Design review of the part built by this model. Coordinates are the model's own, in mm. Face numbers are marked on the shaded views. A direction names the side the tool comes from. Round coordinates to 2 decimals unless told otherwise and drop trailing zeros. Order: outer loops, then holes, each group sorted by start corner. A loop starts at its lowest first (then second) coordinate and runs counter-clockwise, first axis right, second up.
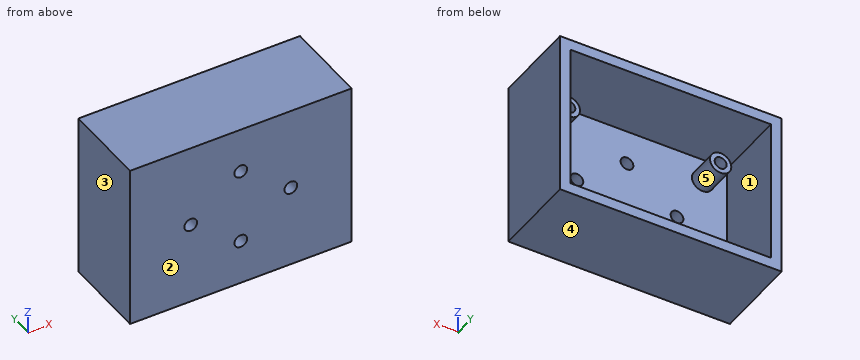
from build123d import *

# Parameters (mm, degrees)
SKETCH_1_W          = 52
SKETCH_1_H          = 39
SKETCH_1_W_2        = 47
SKETCH_1_H_2        = 34
EXTRUDE_1_DEPTH     = 20
SKETCH_2_R          = 2.5
EXTRUDE_2_DEPTH     = 10
EXTRUDE_2_2_DEPTH   = 10
EXTRUDE_2_3_DEPTH   = 10
EXTRUDE_2_4_DEPTH   = 10
SKETCH_3_R          = 1.4
CUT_EXTRUDE_1_DEPTH = 7
SKETCH_4_W          = 52
SKETCH_4_H          = 39
EXTRUDE_3_DEPTH     = 3
SKETCH_5_R          = 1.5
CUT_EXTRUDE_2_DEPTH = 37.67764987


with BuildPart() as part:
    # Sketch 1 → Extrude 1 (new body)
    with BuildSketch(Plane(origin=(0, 0, 0), x_dir=(1, 0, 0), z_dir=(0, 1, 0))):
        Rectangle(SKETCH_1_W, SKETCH_1_H)
        Rectangle(SKETCH_1_W_2, SKETCH_1_H_2, mode=Mode.SUBTRACT)
    extrude(amount=EXTRUDE_1_DEPTH)



with BuildPart() as body_2:
    # Sketch 2 → Extrude 2 (new body)
    with BuildSketch(Plane.XZ):
        with Locations(Location((-17.75, 11.5, 0), (0, 0, 270))):
            Circle(SKETCH_2_R)
    extrude(amount=-EXTRUDE_2_DEPTH)


with BuildPart() as body_3:
    # Sketch 2 → Extrude 2 2 (new body)
    with BuildSketch(Plane.XZ):
        with Locations(Location((17.75, 11.5, 0), (0, 0, 270))):
            Circle(SKETCH_2_R)
    extrude(amount=-EXTRUDE_2_2_DEPTH)


with BuildPart() as body_4:
    # Sketch 2 → Extrude 2 3 (new body)
    with BuildSketch(Plane.XZ):
        with Locations(Location((-17.75, -11.5, 0), (0, 0, 270))):
            Circle(SKETCH_2_R)
    extrude(amount=-EXTRUDE_2_3_DEPTH)


with BuildPart() as body_5:
    # Sketch 2 → Extrude 2 4 (new body)
    with BuildSketch(Plane.XZ):
        with Locations(Location((17.75, -11.5, 0), (0, 0, 270))):
            Circle(SKETCH_2_R)
    extrude(amount=-EXTRUDE_2_4_DEPTH)


with BuildPart() as cut_extrude_1_tool:
    # Sketch 3 → Cut-Extrude 1 (new body)
    with BuildSketch(Plane(origin=(0, 10, 0), x_dir=(1, 0, 0), z_dir=(0, 1, 0))):
        with Locations(Location((-17.75, 11.5, 0), (0, 0, 270))):
            Circle(SKETCH_3_R)
        with Locations(Location((17.75, 11.5, 0), (0, 0, 270))):
            Circle(SKETCH_3_R)
        with Locations(Location((-17.75, -11.5, 0), (0, 0, 270))):
            Circle(SKETCH_3_R)
        with Locations(Location((17.75, -11.5, 0), (0, 0, 270))):
            Circle(SKETCH_3_R)
    extrude(amount=-CUT_EXTRUDE_1_DEPTH)


with BuildPart() as body_2_1:
    add(body_2.part)

    # Cut-Extrude 1: cut by cut_extrude_1_tool
    add(cut_extrude_1_tool.part, mode=Mode.SUBTRACT)


with BuildPart() as body_3_1:
    add(body_3.part)

    # Cut-Extrude 1: cut by cut_extrude_1_tool
    add(cut_extrude_1_tool.part, mode=Mode.SUBTRACT)


with BuildPart() as body_4_1:
    add(body_4.part)

    # Cut-Extrude 1: cut by cut_extrude_1_tool
    add(cut_extrude_1_tool.part, mode=Mode.SUBTRACT)


with BuildPart() as body_5_1:
    add(body_5.part)

    # Cut-Extrude 1: cut by cut_extrude_1_tool
    add(cut_extrude_1_tool.part, mode=Mode.SUBTRACT)


with BuildPart() as part_1:
    add(part.part)

    add(body_2_1.part)  # Extrude 3 merges body 2

    add(body_3_1.part)  # Extrude 3 merges body 3

    add(body_4_1.part)  # Extrude 3 merges body 4

    add(body_5_1.part)  # Extrude 3 merges body 5
    # Sketch 4 → Extrude 3 (add)
    with BuildSketch(Plane.XZ):
        Rectangle(SKETCH_4_W, SKETCH_4_H)
    extrude(amount=-EXTRUDE_3_DEPTH)

    # Sketch 5 → Cut-Extrude 2 (cut, through all)
    with BuildSketch(Plane(origin=(0, 3, 0), x_dir=(1, 0, 0), z_dir=(0, 1, 0))):
        with Locations(Location((0, 8.872353491, 0), (0, 0, 270))):
            Circle(SKETCH_5_R)
        with Locations(Location((11.75, 0, 0), (0, 0, 270))):
            Circle(SKETCH_5_R)
        with Locations(Location((0, -8.872353491, 0), (0, 0, 90))):
            Circle(SKETCH_5_R)
        with Locations(Location((-11.75, 0, 0), (0, 0, 90))):
            Circle(SKETCH_5_R)
    extrude(amount=-CUT_EXTRUDE_2_DEPTH, mode=Mode.SUBTRACT)


solid = part_1.part
1) Take a section at A-A on y = 4.25. State how many separate pieces and enclosed holes the cut face has, plus the area to 3 significant figures.
Results:
separate pieces: 5
enclosed holes: 5
area: 484 mm2
2) Clearance check with flat-ended pins moving along their axes: P1, Ø0.8, axis at x = -17.5, z = 11.5, coming from the +Y side; P2, Ø3.5, axis at x = -17.75, z = 11.5, coming from the +Y side; P3, Ø2.5, axis at x = 0, z = 8.87, coming from the +Y side. State where each tip first meets the part, or that it passes through.
Results:
P1: stops at y = 3
P2: stops at y = 10
P3: passes through
3) The part is to be moulded in two halves that separate along X. For the marked faces 1, 2 and 3, say which applies: released by +X, released by -X, zero draft, split by the parting line, or undercut.
Results:
face 1: undercut
face 2: zero draft
face 3: released by -X
4) To check wall thickness, follow line 1 along X through (y, z) = (4.5, -11.5); line 2 along X through (y, z) = (6.75, -1); line 3 along Z through (x, y) = (-16, 13.75). State the ranges of each line that lie inside material, in increasing order.
Results:
line 1: x = -26 to -23.5, -20.25 to -19.15, -16.35 to -15.25, 15.25 to 16.35, 19.15 to 20.25, 23.5 to 26
line 2: x = -26 to -23.5, 23.5 to 26
line 3: z = -19.5 to -17, 17 to 19.5
5) Take a section at B-B on x = 0. Give the boundary of the cut face in (y, z).
Results:
outline: (0, -19.5) - (20, -19.5) - (20, -17) - (3, -17) - (3, -10.37) - (0, -10.37) - close; (0, -7.37) - (3, -7.37) - (3, 7.37) - (0, 7.37) - close; (0, 10.37) - (3, 10.37) - (3, 17) - (20, 17) - (20, 19.5) - (0, 19.5) - close
6) Take a section at C-C on z = 0. Give the boundary of the cut face in (x, y), plus the area to 3 significant figures.
Results:
outline: (-26, 0) - (-13.25, 0) - (-13.25, 3) - (-23.5, 3) - (-23.5, 20) - (-26, 20) - close; (-10.25, 0) - (10.25, 0) - (10.25, 3) - (-10.25, 3) - close; (13.25, 0) - (26, 0) - (26, 20) - (23.5, 20) - (23.5, 3) - (13.25, 3) - close
area: 223 mm2
7) Take a section at D-D on x = 11.75. Give the boundary of the cut face in (y, z).
Results:
outline: (0, -19.5) - (20, -19.5) - (20, -17) - (3, -17) - (3, -1.5) - (0, -1.5) - close; (0, 1.5) - (3, 1.5) - (3, 17) - (20, 17) - (20, 19.5) - (0, 19.5) - close
8) For the marked faces 4 and 5, list the 3-axis set-ups (+Z, -Z, +X, -X, +Y, -Y) from which the entire face can be reached by the end or side of a thin tool; tool diameter is ignored.
Results:
face 4: -Z, +X, -X, +Y, -Y
face 5: +Y
